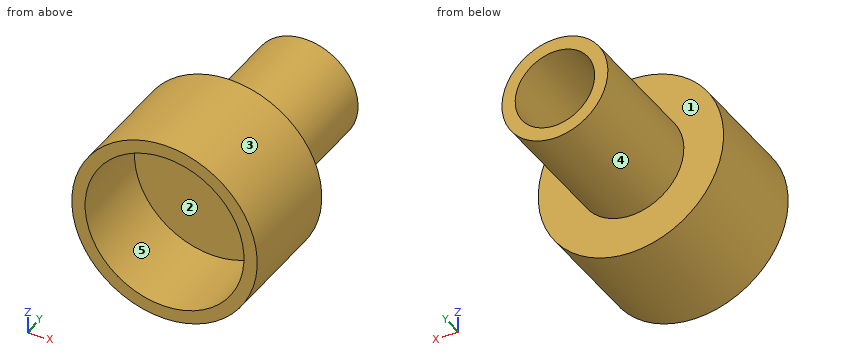
from build123d import *

# Parameters (mm, degrees)
SKETCH1_R           = 4
SKETCH1_R_2         = 3
BOSS_EXTRUDE1_DEPTH = 10
SKETCH2_R           = 7
BOSS_EXTRUDE2_DEPTH = 8.5
SKETCH3_R           = 6
CUT_EXTRUDE1_DEPTH  = 6.5


with BuildPart() as part:
    # Sketch1 → Boss-Extrude1 (new body)
    with BuildSketch(Plane(origin=(0, 0, 0), x_dir=(1, 0, 0), z_dir=(0, 1, 0))):
        with Locations(Location((0, 0, 0), (0, 0, 270))):
            Circle(SKETCH1_R)
        with Locations(Location((0, 0, 0), (0, 0, 270))):
            Circle(SKETCH1_R_2, mode=Mode.SUBTRACT)
    extrude(amount=BOSS_EXTRUDE1_DEPTH)

    # Sketch2 → Boss-Extrude2 (add)
    with BuildSketch(Plane(origin=(0, 0, 0), x_dir=(1, 0, 0), z_dir=(0, 1, 0))):
        with Locations(Location((0, 0, 0), (0, 0, 270))):
            Circle(SKETCH2_R)
    extrude(amount=-BOSS_EXTRUDE2_DEPTH)

    # Sketch3 → Cut-Extrude1 (cut)
    with BuildSketch(Plane.XZ.offset(8.5)):
        with Locations(Location((0, 0, 0), (0, 0, 270))):
            Circle(SKETCH3_R)
    extrude(amount=-CUT_EXTRUDE1_DEPTH, mode=Mode.SUBTRACT)


solid = part.part
Could you check a few things on this model? Use its own coordinates, in mm. Face numbers are marked on the shaded views. A direction names the side the tool comes from. Coordinates: 2 decimals unless noted, no trailing zeros. Write each loop counter-clockwise with the first axis right and the second up, starting at its lowest first coordinate (ties: lowest second). Pieces come first, ordered by that corner, then holes. Notation, with made-up numbers: (70.25, 0.25) - (109.25, 0.25) arc R22 cw to (109.25, 20.25) - close; hole circle Ø10 at (88.5, 27). An arc over 180 degrees is marked (long way). Put each result on its own line as item: value. Start each with the question number.
Q1. I want a section at A-A on x = 0. Write out the boundary of the cut face in (y, z).
Q2. Thinking about a two-plate mould opening in Z: for the marked faces 1, 2 and 3, which applies, pulls with the +Z half, pulls with the -Z half, needs draft (parallel to the pull), parting line crosses it, or undercut?
Q3. Which directions (+Z, -Z, +X, -X, +Y, -Y) give clear straight access to the entire face, cutting with the end or side of a thin tool? Please do the marked faces 4 and 5.
Q4. I want a section at C-C on y = 1.5. Write out the boundary of the cut face in (x, z).
Q5. Please list where these lines run through material, in increasing order: L1, parallel to Y at x = 2.5, z = -4; L2, parallel to Y at x = -4.5, z = -4.5; L3, parallel to X at y = -2.75, z = -4.
Q6. I want a section at B-B on z = 0. Write out the boundary of the cut face in (x, y), plus the area to 3 significant figures.
Q7. I want a section at D-D on x = 4.5. Write out the boundary of the cut face in (y, z), plus the area to 3 significant figures.
Q8. I'm going to push flat-ended pins straight in: P1, Ø1.5, axis at x = 1, z = 0.5, coming from the +Y side; P2, Ø2, axis at y = -2, z = -3.5, coming from the -X side; P3, Ø8, axis at x = -1.5, z = 0.5, coming from the -Y side; P4, Ø4, axis at x = 3, z = 3, coming from the +Y side. Where does each tip first touch, or does it pass through?
Checks:
1. outline: (-8.5, -7) - (0, -7) - (0, -4) - (10, -4) - (10, -3) - (0, -3) - (0, 3) - (10, 3) - (10, 4) - (0, 4) - (0, 7) - (-8.5, 7) - (-8.5, 6) - (-2, 6) - (-2, -6) - (-8.5, -6) - close
2. face 1: needs draft
2. face 2: undercut
2. face 3: parting line crosses it
3. face 4: +Y
3. face 5: -Y
4. outline: circle Ø8 at (0, 0); hole circle Ø6 at (0, 0)
5. L1: -2 to 0
5. L2: -8.5 to 0
5. L3: -5.74 to -4.47, 4.47 to 5.74
6. outline: (-7, -8.5) - (-6, -8.5) - (-6, -2) - (6, -2) - (6, -8.5) - (7, -8.5) - (7, 0) - (4, 0) - (4, 10) - (3, 10) - (3, 0) - (-3, 0) - (-3, 10) - (-4, 10) - (-4, 0) - (-7, 0) - close
6. area: 61.0 mm²
7. outline: (-8.5, -5.36) - (0, -5.36) - (0, 5.36) - (-8.5, 5.36) - (-8.5, 3.97) - (-2, 3.97) - (-2, -3.97) - (-8.5, -3.97) - close
7. area: 39.6 mm²
8. P1: y = 0
8. P2: x = -6.54
8. P3: y = -2
8. P4: y = 10
